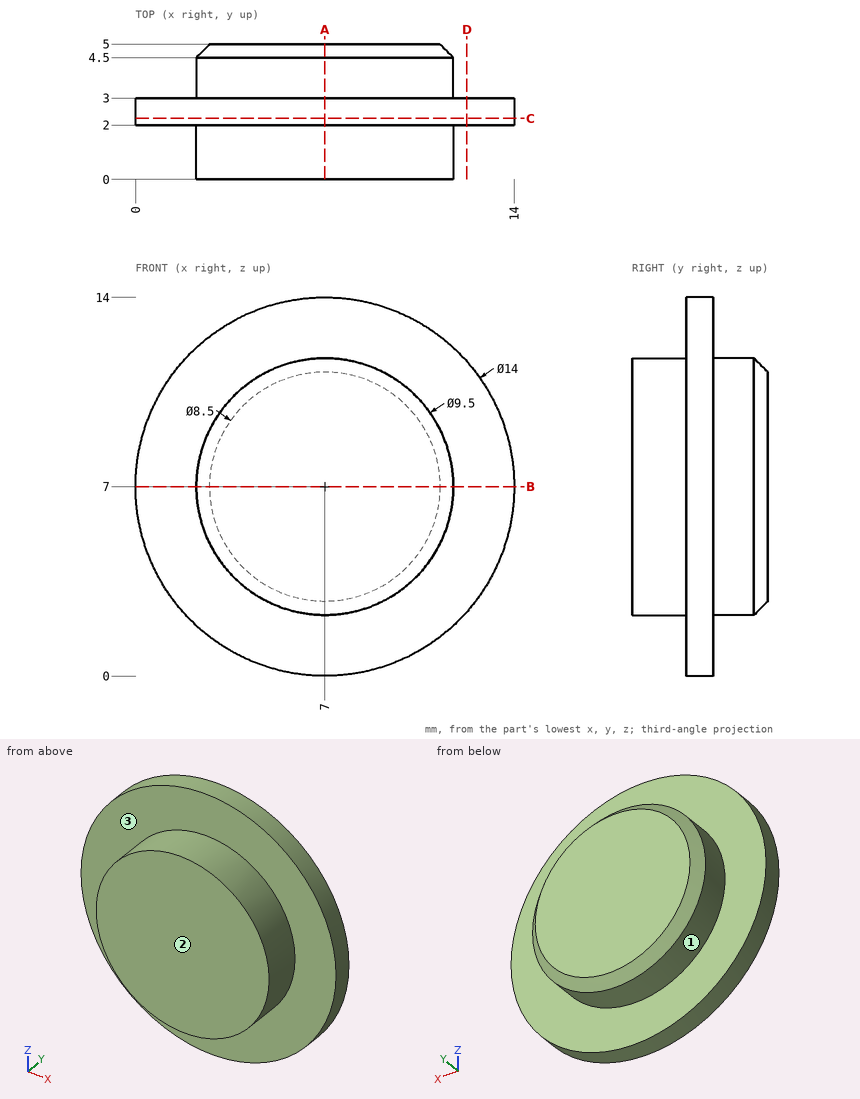
The figure shows three views and two pictorial views of one solid part (mm, origin at its lowest corner). Answer the questions. A direction names the side the tool comes from. Give positions to 0.01 mm unless a question says otherwise; leave off trailing zeros. Loops run counter-clockwise (first coordinate to the right, second up) from the corner with the lowest first, then second, coordinate; pieces in that order, holes last. Notation, with made-up numbers: M 48.25,-15 L 96.25,-15 A14 cw 96.25,10 Z; hole C 82,16 d8. An arc over 180 degrees is marked long. Write each question's results on one line, items separated by ' | '.
1. Section C-C on y = 2.25 is taken. Give the vertices of the cut face in (x, z).
Values:
outline: C 7,7 d14
2. A tool of negligible diameter and unlimited length cuts with its end or side. For the marked faces 1, 2 and 3, from which of +Z, -Z, +X, -X, +Y, -Y can it reach the whole face along a straight path? Write none if from no direction.
Values:
face 1: +Y | face 2: +Z, -Z, +X, -X, -Y | face 3: -Y
3. Section B-B on z = 7 is taken. Give the vertices of the cut face in (x, y), plus the area to 4 significant figures.
Values:
outline: M 0,2 L 2.25,2 L 2.25,0 L 11.75,0 L 11.75,2 L 14,2 L 14,3 L 11.75,3 L 11.75,4.5 L 11.25,5 L 2.75,5 L 2.25,4.5 L 2.25,3 L 0,3 Z | area: 51.75 mm^2
4. Straight lines are drawn through the part: line 1 (Y direction, x = 2, z = 5); line 2 (Z direction, x = 3.25, y = 0.65); line 3 (X direction, y = 3.35, z = 9.5). For each, find the intervals that lie inside material, in ascending order. Write a range as [from, to].
Values:
line 1: y = [2, 3] | line 2: z = [4.08, 9.92] | line 3: x = [2.96, 11.04]
5. Section A-A on x = 7 is taken. Give the vertices of the cut face in (y, z), plus the area to 4 significant figures.
Values:
outline: M 0,2.25 L 2,2.25 L 2,0 L 3,0 L 3,2.25 L 4.5,2.25 L 5,2.75 L 5,11.25 L 4.5,11.75 L 3,11.75 L 3,14 L 2,14 L 2,11.75 L 0,11.75 Z | area: 51.75 mm^2
6. Given pin 1 (8 mm diameter, centred on x = 1.5, z = 6.5, fed in from -Y); pin 2 (1.5 mm diameter, centred on x = 12.5, z = 8.5, fed in from -Y), each flat-ended and moving along its own axis, determine where each tip first touches the part or whether it passes through.
Values:
pin 1: stops at y = 0 | pin 2: stops at y = 2
7. Section D-D on x = 12.25 is taken. Give the vertices of the cut face in (y, z), plus the area to 3 significant figures.
Values:
outline: M 2,2.37 L 3,2.37 L 3,11.63 L 2,11.63 Z | area: 9.26 mm^2
